Autodesk Inventor part; units mm, degrees
ref_plane "YZ Plane" through (0, 0, 0) normal (1, 0, 0) x (0, 1, 0)
ref_plane "XZ Plane" through (0, 0, 0) normal (0, 1, 0) x (-1, 0, 0)
ref_plane "XY Plane" through (0, 0, 0) normal (0, 0, 1) x (1, 0, 0)
sketch "Sketch1" plane through (0, 0, 0) normal (0, 0, 1) x (1, 0, 0)
  line L0 (40, 28.5) -> (-40, 28.5)
  line L1 (-40, 28.5) -> (-40, -28.5)
  line L2 (-40, -28.5) -> (40, -28.5)
  line L3 (40, -28.5) -> (40, 28.5)
  line L4 (40, 28.5) -> (-40, -28.5) construction
  line L5 (-40, 28.5) -> (40, -28.5) construction
  line L6 (-33, 24.25) -> (33, 24.25) construction
  line L7 (33, 24.25) -> (33, -24.25) construction
  line L8 (33, -24.25) -> (-33, -24.25) construction
  line L9 (-33, -24.25) -> (-33, 24.25) construction
  line L10 (-33, 24.25) -> (33, -24.25) construction
  line L11 (33, 24.25) -> (-33, -24.25) construction
  line L12 (40, 0) -> (-40, 0) construction
  line L13 (0, 28.5) -> (0, -28.5) construction
  circle A0 centre (33, 24.25) radius 2.4
  circle A1 centre (-33, 24.25) radius 2.4
  circle A2 centre (33, -24.25) radius 2.4
  circle A3 centre (-33, -24.25) radius 2.4
  line L14 (33, 27.5) -> (33, 21) construction
  arc A4 (32.2801, 21.9605) -> (33.7199, 21.9605) centre (33, 21.75) ccw
  arc A5 (-33.7199, 21.9605) -> (-32.2801, 21.9605) centre (-33, 21.75) ccw
  arc A6 (33.7199, -21.9605) -> (32.2801, -21.9605) centre (33, -21.75) ccw
  arc A7 (-32.2801, -21.9605) -> (-33.7199, -21.9605) centre (-33, -21.75) ccw
  line L15 (39, 20) -> (-39, 20)
  line L16 (-39, 20) -> (-39, -20)
  line L17 (-39, -20) -> (39, -20)
  line L18 (39, -20) -> (39, 20)
  line L19 (39, 20) -> (-39, -20) construction
  line L20 (-39, 20) -> (39, -20) construction
  arc A8 (33.7199, 26.5395) -> (32.2801, 26.5395) centre (33, 26.75) ccw
  arc A9 (-32.2801, 26.5395) -> (-33.7199, 26.5395) centre (-33, 26.75) ccw
  arc A10 (32.2801, -26.5395) -> (33.7199, -26.5395) centre (33, -26.75) ccw
  arc A11 (-33.7199, -26.5395) -> (-32.2801, -26.5395) centre (-33, -26.75) ccw
  point P0 (0, 0)
  point P1 (33, -21)
  point P2 (-32.2801, 21.9605)
  point P3 (-33.7199, 21.9605)
  point P4 (-33.7199, -21.9605)
  point P5 (-32.2801, -21.9605)
  point P6 (32.2801, -21.9605)
  point P7 (33.7199, -21.9605)
  point P8 (32.2801, 26.5395)
  point P9 (33.7199, 26.5395)
  point P10 (-33.7199, 26.5395)
  point P11 (-32.2801, 26.5395)
  point P12 (-32.2801, -26.5395)
  point P13 (-33.7199, -26.5395)
  point P14 (33.7199, -26.5395)
  point P15 (32.2801, -26.5395)
  dimension "d0" = 80
  dimension "d1" = 57
  dimension "d19" = 4.8
  dimension "d30" = 6.5
  dimension "d33" = 48.5
  dimension "d34" = 66
  dimension "d36" = 1.5
  dimension "d37" = 8.5
  dimension "d38" = 1
  dimension "d41" = 14
  dimension "d42" = 6.5
  dimension "d43" = 1
extrude "Extrusion1" add sketch "Sketch1" along normal blind 1.6 contours L3 L2 L1 L0 | L18 L17 L16 L15
extrude "Extrusion2" add sketch "Sketch1" along normal blind 16.6 contours L18 L17 L16 L15
fillet "Fillet1" radius 2 4 edges at (39, -20, 9.1) (39, 20, 9.1) (-39, -20, 9.1) (-39, 20, 9.1)
properties part number "SUSTAINA-POWER-DISTRIBUTION-BOARD" material "Acetal Resin, Black"
For this review, take the finished solid that the model builds, in its own axes (mm). A direction names the side the tool comes from. Round coordinates to 2 decimals unless told otherwise and drop trailing zeros. Loops run counter-clockwise (first coordinate to the right, second up) from the corner with the lowest first, then second, coordinate; pieces in that order, holes last. Notation, with made-up numbers: (33.25, -29) - (49.25, -29) arc R21 ccw to (49.25, -8) - close; hole circle Ø11 at (16.5, -31). An arc over 180 degrees is marked (long way). Use one line per item in the form item = value.
1) Tool access review of faces 1 (the face through (-39, 0, 9)), 2 (the face through (-1, -20, 9)), 3 (the face through (39, 0, 9)), 4 (the face through (-30.6, 24.3, 0.8)), 5 (the face through (-1, 0, 16.6)): name each direction out of +Z, -Z, +X, -X, +Y, -Y from which nothing blocks a thin tool from reaching the whole face with its end or side.
Solutions:
face_1 = +Z, -X, +Y, -Y
face_2 = +Z, +X, -X, -Y
face_3 = +Z, +X, +Y, -Y
face_4 = +Z, -Z
face_5 = +Z, +X, -X, +Y, -Y
2) We need section C-C on y = 25. Write out the cut boundary in (x, z), then the cut area to 3 significant figures.
Solutions:
outline = (-40, 0) - (-35.28, 0) - (-35.28, 1.6) - (-40, 1.6) - close; (-30.72, 0) - (30.72, 0) - (30.72, 1.6) - (-30.72, 1.6) - close; (35.28, 0) - (40, 0) - (40, 1.6) - (35.28, 1.6) - close
area = 113 mm2
3) Wall thickness on probe 1 along X at (y, z) = (-26.75, 1); probe 2 along X at (y, z) = (23, 1); probe 3 along Z at (x, y) = (11.5, 26.5): over which ranges is each line inside the solid? List them lowest first.
Solutions:
probe_1 = -40 to -33.75, -32.25 to 32.25, 33.75 to 40
probe_2 = -40 to -35.05, -30.95 to 30.95, 35.05 to 40
probe_3 = 0 to 1.6
4) We need section B-B on x = -3.5. Write out the cut boundary in (y, z), then the cut area to 3 significant figures.
Solutions:
outline = (-28.5, 0) - (28.5, 0) - (28.5, 1.6) - (20, 1.6) - (20, 16.6) - (-20, 16.6) - (-20, 1.6) - (-28.5, 1.6) - close
area = 691 mm2
5) Clearance check with flat-ended pins moving along their axes: P1, Ø2.5, axis at x = 33, y = 21.75, coming from the +Z side; P2, Ø6, axis at x = -19, z = 6.5, coming from the -Y side; P3, Ø1.4, axis at x = 33, y = -21.75, coming from the +Z side; P4, Ø3, axis at y = 5, z = 7.5, coming from the +X side. State where each tip first meets the part, or that it passes through.
Solutions:
P1 = 1.6
P2 = -20
P3 = through
P4 = 39
6) Mouldability with a two-part tool opening along X and no side actions: class faces 6 (the face through (38.4, -19.43, 9.21)), 7 (the face through (-38.43, -19.4, 9.21)), 8 (the face through (-30.6, -24.2, 0.8)), 9 (the face through (1, 20, 9)) as pulls with the +X half, pulls with the -X half, needs draft (parallel to the pull), parting line crosses it, or undercut.
Solutions:
face_6 = pulls with the +X half
face_7 = pulls with the -X half
face_8 = undercut
face_9 = needs draft
7) We need section A-A on z = 7.25. Write out the cut boundary in (x, y), then the cut area to 3 significant figures.
Solutions:
outline = (-39, -18) arc R2 ccw to (-37, -20) - (37, -20) arc R2 ccw to (39, -18) - (39, 18) arc R2 ccw to (37, 20) - (-37, 20) arc R2 ccw to (-39, 18) - close
area = 3,120 mm2
